Design review of the part shown in the three views and the two pictorial views. Dimensions are in mm from the part's minimum x, y and z. Give positions to 0.01 mm unless a question says otherwise; leave off trailing zeros. Order: outer loops, then holes, each group sorted by start corner. A loop starts at its lowest first (then second) coordinate and runs counter-clockwise, first axis right, second up.
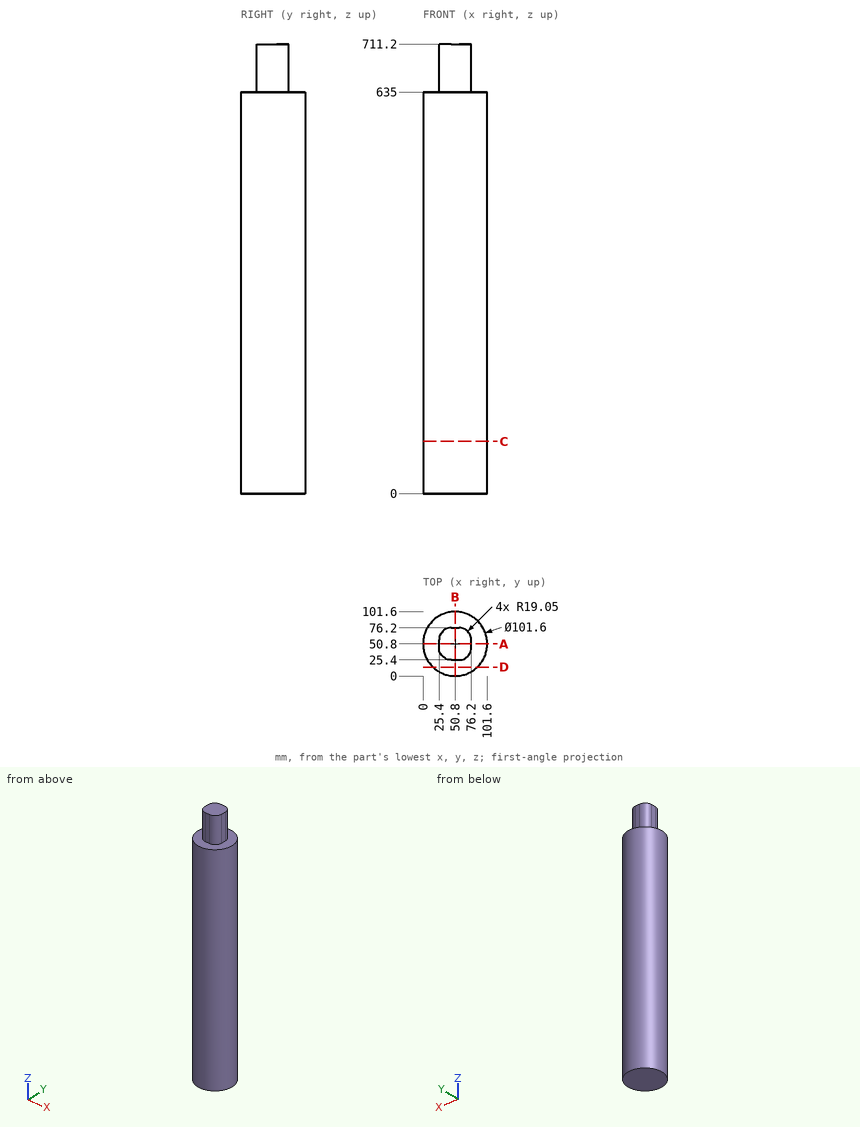
1) Clearance check with flat-ended pins moving along their axes: pin 1 (5 mm diameter, centred on x = 78, z = 230.5, fed in from +Y); pin 2 (14 mm diameter, centred on x = 51.5, z = 680, fed in from -Y); pin 3 (10 mm diameter, centred on y = 90.5, z = 639, fed in from -X); pin 4 (4 mm diameter, centred on x = 77.5, y = 55.5, fed in from -Z). State where each tip first meets the part, or that it passes through.
Answer sheet:
pin 1: stops at y = 95.19
pin 2: stops at y = 25.4
pin 3: stops at x = 15.68
pin 4: stops at z = 0
2) To check wall thickness, follow line 1 (X direction, y = 57.5, z = 681); line 2 (Z direction, x = 66, y = 78); line 3 (X direction, y = 48, z = 483). State the ranges of each line that lie inside material, in increasing order.
Answer sheet:
line 1: x = 25.4 to 76.2
line 2: z = 0 to 635
line 3: x = 0.08 to 101.52
3) We need section A-A on y = 50.8. Give the boundary of the cut face in (x, z), then the cut area to 3 significant figures.
Answer sheet:
outline: (0, 0) - (101.6, 0) - (101.6, 635) - (76.2, 635) - (76.2, 711.2) - (25.4, 711.2) - (25.4, 635) - (0, 635) - close
area: 68,400 mm2
4) We need section C-C on z = 83. Give the boundary of the cut face in (x, y).
Answer sheet:
outline: circle Ø101.6 at (50.8, 50.8)
5) We need section D-D on y = 14. Give the boundary of the cut face in (x, z).
Answer sheet:
outline: (15.78, 0) - (85.82, 0) - (85.82, 635) - (15.78, 635) - close
